Here's how the part is built. I have some questions about the finished solid (model axes, mm). Face numbers are marked on the shaded views. A direction names the side the tool comes from. Give positions to 0.01 mm unless a question says otherwise; leave off trailing zeros. Loops run counter-clockwise (first coordinate to the right, second up) from the corner with the lowest first, then second, coordinate; pieces in that order, holes last.
Q1. I'm going to push flat-ended pins straight in: P1, Ø10, axis at x = -1.5, z = -2.5, coming from the -Y side; P2, Ø12, axis at y = 163.5, z = 49.5, coming from the +X side; P3, Ø6, axis at x = 9.5, y = 16.5, coming from the -Z side. Where does each tip first touch, or does it pass through?
Q2. Suppose I cut it at D-D (x = 33). List the corners of the cut face in (y, z) for me.
Q3. Suppose I cut it at B-B (z = 8.5). Count the separate pieces of the cut face and the enclosed holes in it, and give its area (3 significant figures).
Q4. Suppose I cut it at C-C (y = 20.5). List the corners of the cut face in (x, z) for me, and give its area (3 significant figures).
Q5. I need wall thicknesses on probe 1 along X at (y, z) = (172, 0); probe 2 along Y at (x, z) = (-16, -13.5); probe 3 along Z at (x, y) = (1, 4) (1 decimal). Which ranges of each line are inside material? Lowest first, please.
Q6. Thinking about a two-plate mould opening in X: for the marked faces 1, 2 and 3, which applies, pulls with the +X half, pulls with the -X half, needs draft (parallel to the pull), parting line crosses it, or undercut?
Q7. Suppose I cut it at A-A (y = 195). List the corners of the cut face in (x, z) for me, and give its area (3 significant figures).
Q8. For the marked faces 4, 5 and 6, which set-ups out of +Z, -Z, +X, -X, +Y, -Y let a thin tool reach every point of the face, with its end or its side?
```python
from build123d import *

# Parameters (mm, degrees)
CROQUIS1_R               = 40
CROQUIS1_R_2             = 6
SALIENTE_EXTRUIR1_DEPTH  = 30
SALIENTE_EXTRUIR2_START  = 20
CROQUIS2_R               = 40
CROQUIS2_R_2             = 35.3
SALIENTE_EXTRUIR2_DEPTH  = 20
CROQUIS6_R               = 6
CORTAR_EXTRUIR3_DEPTH    = 25
CROQUIS7_R               = 25
CROQUIS7_R_2             = 21
SALIENTE_EXTRUIR3_DEPTH  = 140
CROQUIS9_W               = 50
CROQUIS9_H               = 50
CROQUIS9_R               = 6
SALIENTE_EXTRUIR4_DEPTH  = 5
CROQUIS17_W              = 40
CROQUIS17_H              = 50
SALIENTE_EXTRUIR9_DEPTH  = 40
CROQUIS18_W              = 58.160908148
CROQUIS18_H              = 40
SALIENTE_EXTRUIR10_DEPTH = 40
REDONDEO1_R              = 3
CROQUIS19_R              = 12.65
CROQUIS19_R_2            = 4.5
CORTAR_EXTRUIR7_DEPTH    = 40
CROQUIS20_R              = 12.15
CORTAR_EXTRUIR8_DEPTH    = 8
CORTAR_EXTRUIR9_START    = -8
CROQUIS21_R              = 12.15
CORTAR_EXTRUIR9_DEPTH    = 8
SALIENTE_EXTRUIR11_DEPTH = 40


with BuildPart() as part:
    # Croquis1 → Saliente-Extruir1 (new body)
    with BuildSketch(Plane(origin=(0, 0, 0), x_dir=(1, 0, 0), z_dir=(0, 1, 0))):
        with Locations(Location((0, 0, 0), (0, 0, 270))):
            Circle(CROQUIS1_R)
        with Locations(Location((0, 0, 0), (0, 0, 270))):
            Circle(CROQUIS1_R_2, mode=Mode.SUBTRACT)
    extrude(amount=SALIENTE_EXTRUIR1_DEPTH)

    # Croquis2 → Saliente-Extruir2 (add)
    with BuildSketch(Plane.XZ.offset(SALIENTE_EXTRUIR2_START)):
        with Locations(Location((0, 0, 0), (0, 0, 270))):
            Circle(CROQUIS2_R)
        with Locations(Location((0, 0, 0), (0, 0, 270))):
            Circle(CROQUIS2_R_2, mode=Mode.SUBTRACT)
    extrude(amount=-SALIENTE_EXTRUIR2_DEPTH)

    # Croquis6 → Cortar-Extruir3 (cut)
    with BuildSketch(Plane.XZ):
        Polygon((-3.453364776, -6.205181039), (3.647162027, -6.093292144), (7.100526803, 0.111888895), (3.453364776, 6.205181039), (-3.647162027, 6.093292144), (-7.100526803, -0.111888895), align=None)
        with Locations(Location((0, 0, 0), (0, 0, 270))):
            Circle(CROQUIS6_R, mode=Mode.SUBTRACT)
    extrude(amount=-CORTAR_EXTRUIR3_DEPTH, mode=Mode.SUBTRACT)

    # Croquis7 → Saliente-Extruir3 (add)
    with BuildSketch(Plane(origin=(0, 30, 0), x_dir=(1, 0, 0), z_dir=(0, 1, 0))):
        with Locations(Location((0, 0, 0), (0, 0, 270))):
            Circle(CROQUIS7_R)
        with Locations(Location((0, 0, 0), (0, 0, 270))):
            Circle(CROQUIS7_R_2, mode=Mode.SUBTRACT)
    extrude(amount=SALIENTE_EXTRUIR3_DEPTH)

    # Croquis9 → Saliente-Extruir4 (add)
    with BuildSketch(Plane(origin=(0, 170, 0), x_dir=(1, 0, 0), z_dir=(0, 1, 0))):
        Rectangle(CROQUIS9_W, CROQUIS9_H)
        with Locations(Location((0, 0, 0), (0, 0, 90))):
            Circle(CROQUIS9_R, mode=Mode.SUBTRACT)
    extrude(amount=SALIENTE_EXTRUIR4_DEPTH)

    # Croquis17 → Saliente-Extruir9 (add)
    with BuildSketch(Plane(origin=(0, 175, 0), x_dir=(1, 0, 0), z_dir=(0, 1, 0))):
        Rectangle(CROQUIS17_W, CROQUIS17_H)
    extrude(amount=SALIENTE_EXTRUIR9_DEPTH)

    # Croquis18 → Saliente-Extruir10 (add)
    with BuildSketch(Plane.ZY.offset(20)):
        with Locations((54.080454074, 195)):
            Rectangle(CROQUIS18_W, CROQUIS18_H)
    extrude(amount=-SALIENTE_EXTRUIR10_DEPTH)

    # Redondeo1
    # the kernel refuses this fillet: 3 mm, written as the material it takes off along each edge
    with BuildSketch(Plane(origin=(-20, 175, 25), x_dir=(1, 0, 0), z_dir=(0, 0, 1)), Plane(origin=(20, 215, 90.660908148), x_dir=(0, -1, 0), z_dir=(0, 0, -1))) as redondeo1_piece_1:
        with BuildLine():
            CenterArc((REDONDEO1_R, REDONDEO1_R), REDONDEO1_R, 180, 90)
            Line((0, REDONDEO1_R), (0, 0))
            Line((0, 0), (REDONDEO1_R, 0))
        make_face()
    extrude(amount=65.660908148, mode=Mode.SUBTRACT)
    with BuildSketch(Plane(origin=(20, 175, 25), x_dir=(-1, 0, 0), z_dir=(0, 0, 1)), Plane(origin=(-20, 215, 90.660908148), x_dir=(0, -1, 0), z_dir=(0, 0, -1))) as redondeo1_piece_2:
        with BuildLine():
            CenterArc((REDONDEO1_R, -REDONDEO1_R), REDONDEO1_R, 90, 90)
            Line((0, -REDONDEO1_R), (0, 0))
            Line((0, 0), (REDONDEO1_R, 0))
        make_face()
    extrude(amount=65.660908148, mode=Mode.SUBTRACT)
    with BuildSketch(Plane(origin=(-20, 167.5, 83.160908148), x_dir=(1, 0, 0), z_dir=(0, 1, 0))) as redondeo1_piece_3:
        with BuildLine():
            CenterArc((REDONDEO1_R, REDONDEO1_R), REDONDEO1_R, 180, 90)
            Line((0, REDONDEO1_R), (0, 0))
            Line((0, 0), (REDONDEO1_R, 0))
        make_face()
    extrude(amount=55, mode=Mode.SUBTRACT)
    with BuildSketch(Plane(origin=(20, 167.5, 83.160908148), x_dir=(-1, 0, 0), z_dir=(0, 1, 0))) as redondeo1_piece_4:
        with BuildLine():
            CenterArc((REDONDEO1_R, -REDONDEO1_R), REDONDEO1_R, 90, 90)
            Line((0, -REDONDEO1_R), (0, 0))
            Line((0, 0), (REDONDEO1_R, 0))
        make_face()
    extrude(amount=55, mode=Mode.SUBTRACT)
    with BuildSketch(Plane(origin=(-20, 175, -25), x_dir=(1, 0, 0), z_dir=(0, 1, 0))) as redondeo1_piece_5:
        with BuildLine():
            CenterArc((REDONDEO1_R, -REDONDEO1_R), REDONDEO1_R, 90, 90)
            Line((0, -REDONDEO1_R), (0, 0))
            Line((0, 0), (REDONDEO1_R, 0))
        make_face()
    extrude(amount=47.5, mode=Mode.SUBTRACT)
    with BuildSketch(Plane(origin=(20, 175, -25), x_dir=(-1, 0, 0), z_dir=(0, 1, 0))) as redondeo1_piece_6:
        with BuildLine():
            CenterArc((REDONDEO1_R, REDONDEO1_R), REDONDEO1_R, 180, 90)
            Line((0, REDONDEO1_R), (0, 0))
            Line((0, 0), (REDONDEO1_R, 0))
        make_face()
    extrude(amount=47.5, mode=Mode.SUBTRACT)
    with BuildSketch(Plane(origin=(20, 215, -32.5), x_dir=(0, -1, 0), z_dir=(0, 0, 1)), Plane(origin=(-20, 215, 25), x_dir=(0, -1, 0), z_dir=(0, 0, -1))) as redondeo1_piece_7:
        with BuildLine():
            CenterArc((REDONDEO1_R, -REDONDEO1_R), REDONDEO1_R, 90, 90)
            Line((0, -REDONDEO1_R), (0, 0))
            Line((0, 0), (REDONDEO1_R, 0))
        make_face()
    extrude(amount=57.5, mode=Mode.SUBTRACT)

    # Croquis19 → Cortar-Extruir7 (cut)
    with BuildSketch(Plane.ZY.offset(20)):
        with Locations((0, 195)):
            Circle(CROQUIS19_R)
        with Locations((58.296529275, 195)):
            Circle(CROQUIS19_R_2)
    extrude(amount=-CORTAR_EXTRUIR7_DEPTH, mode=Mode.SUBTRACT)

    # Croquis20 → Cortar-Extruir8 (cut)
    with BuildSketch(Plane.ZY.offset(20)):
        with Locations((58.296529275, 195)):
            Circle(CROQUIS20_R)
    extrude(amount=-CORTAR_EXTRUIR8_DEPTH, mode=Mode.SUBTRACT)

    # Croquis21 → Cortar-Extruir9 (cut)
    with BuildSketch(Plane(origin=(20, 0, 0), x_dir=(0, 0, -1), z_dir=(1, 0, 0)).offset(CORTAR_EXTRUIR9_START)):
        with Locations(Location((-58.296529275, 195, 0), (0, 0, 180))):
            Circle(CROQUIS21_R)
    extrude(amount=CORTAR_EXTRUIR9_DEPTH, mode=Mode.SUBTRACT)

    # Croquis22 → Saliente-Extruir11 (add)
    with BuildSketch(Plane(origin=(20, 0, 0), x_dir=(0, 0, -1), z_dir=(1, 0, 0))):
        Polygon((-80.160908148, 178), (-13.008016213, 178), (-13.008016213, 87.984326583), align=None)
    extrude(amount=-SALIENTE_EXTRUIR11_DEPTH)


solid = part.part
```
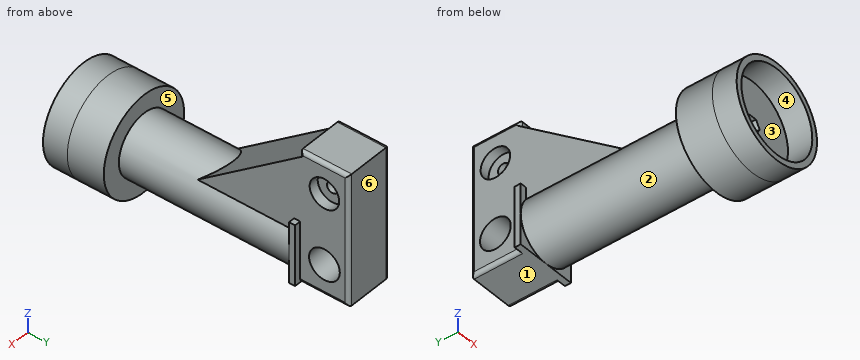
Solutions:
1. P1: stops at y = 0
1. P2: stops at x = 20
1. P3: stops at z = -39.47
2. outline: (-20, -22.61) - (30, -22.61) - (30, 22.61) - (-20, 22.61) - (-20, 12.53) - (0, 12.53) - (0, -12.53) - (-20, -12.53) - close
3. separate pieces: 2
3. enclosed holes: 1
3. area: 4,840 mm2
4. outline: circle Ø80 at (0, 0); hole (-7.1, -0.11) - (-3.45, -6.21) - (3.65, -6.09) - (7.1, 0.11) - (3.45, 6.21) - (-3.65, 6.09) - close
4. area: 4,900 mm2
5. probe 1: x = -25 to -6, 6 to 25
5. probe 2: y = 0 to 30, 170 to 215
5. probe 3: z = -40 to -6.1, 6.2 to 40
6. face 1: needs draft
6. face 2: parting line crosses it
6. face 3: undercut
7. outline: (-20, -22) arc R3 ccw to (-17, -25) - (17, -25) arc R3 ccw to (20, -22) - (20, -12.65) - (-20, -12.65) - close; (-20, 12.65) - (20, 12.65) - (20, 46.15) - (12, 46.15) - (12, 53.8) - (-12, 53.8) - (-12, 46.15) - (-20, 46.15) - close; (-20, 70.45) - (-12, 70.45) - (-12, 62.8) - (12, 62.8) - (12, 70.45) - (20, 70.45) - (20, 80.16) arc R3 ccw to (17, 83.16) - (-17, 83.16) arc R3 ccw to (-20, 80.16) - close
7. area: 2,700 mm2
8. face 4: -Y
8. face 5: none
8. face 6: +Z, -Z, +X, -X, +Y
